from build123d import *

# Parameters (mm, degrees)
SKETCH1_W           = 110
SKETCH1_H           = 84.3
SKETCH1_R           = 1.5
SKETCH1_R_2         = 1.8
BOSS_EXTRUDE1_DEPTH = 3
BOSS_EXTRUDE2_START = 3
SKETCH2_R           = 3
SKETCH2_R_2         = 1.5
BOSS_EXTRUDE2_DEPTH = 3
FILLET1_R           = 3


with BuildPart() as part:
    # Sketch1 → Boss-Extrude1 (new body)
    with BuildSketch(Plane.XY):
        Rectangle(SKETCH1_W, SKETCH1_H)
        with Locations((51, 38.15)):
            Circle(SKETCH1_R, mode=Mode.SUBTRACT)
        with Locations(Location((-51, 38.15, 0), (0, 0, 180))):
            Circle(SKETCH1_R, mode=Mode.SUBTRACT)
        with Locations(Location((51, -38.15, 0), (0, 0, 180))):
            Circle(SKETCH1_R, mode=Mode.SUBTRACT)
        with Locations((-51, -38.15)):
            Circle(SKETCH1_R, mode=Mode.SUBTRACT)
        with Locations((-25, -17.15)):
            Circle(SKETCH1_R_2, mode=Mode.SUBTRACT)
        with Locations((-25, 2.85)):
            Circle(SKETCH1_R_2, mode=Mode.SUBTRACT)
        with Locations((10, 2.85)):
            Circle(SKETCH1_R_2, mode=Mode.SUBTRACT)
        with Locations((10, -17.15)):
            Circle(SKETCH1_R_2, mode=Mode.SUBTRACT)
    extrude(amount=BOSS_EXTRUDE1_DEPTH)

    # Sketch2 → Boss-Extrude2 (add)
    # profile 1 of 4: a face of its own
    with BuildSketch(Plane.XY.offset(BOSS_EXTRUDE2_START)):
        with Locations(Location((-51, 38.15, 0), (0, 0, 180))):
            Circle(SKETCH2_R)
        with Locations(Location((-51, 38.15, 0), (0, 0, 180))):
            Circle(SKETCH2_R_2, mode=Mode.SUBTRACT)
    # profile 2 of 4: a face of its own
    with BuildSketch(Plane.XY.offset(BOSS_EXTRUDE2_START)):
        with Locations(Location((51, 38.15, 0), (0, 0, 180))):
            Circle(SKETCH2_R)
        with Locations(Location((51, 38.15, 0), (0, 0, 180))):
            Circle(SKETCH2_R_2, mode=Mode.SUBTRACT)
    # profile 3 of 4: a face of its own
    with BuildSketch(Plane.XY.offset(BOSS_EXTRUDE2_START)):
        with Locations(Location((51, -38.15, 0), (0, 0, 180))):
            Circle(SKETCH2_R)
        with Locations(Location((51, -38.15, 0), (0, 0, 180))):
            Circle(SKETCH2_R_2, mode=Mode.SUBTRACT)
    # profile 4 of 4: a face of its own
    with BuildSketch(Plane.XY.offset(BOSS_EXTRUDE2_START)):
        with Locations(Location((-51, -38.15, 0), (0, 0, 180))):
            Circle(SKETCH2_R)
        with Locations(Location((-51, -38.15, 0), (0, 0, 180))):
            Circle(SKETCH2_R_2, mode=Mode.SUBTRACT)
    extrude(amount=BOSS_EXTRUDE2_DEPTH)

    # Fillet1
    # the kernel refuses this fillet: 3 mm, written as the material it adds along each edge
    with BuildSketch(Plane(origin=(-51, 38.15, 3), x_dir=(-1, 0, 0), z_dir=(0, 1, 0))) as fillet1_piece_1_section:
        with BuildLine():
            CenterArc((3 + FILLET1_R, FILLET1_R), FILLET1_R, 180, 90)
            Line((3, FILLET1_R), (3, 0))
            Line((3, 0), (3 + FILLET1_R, 0))
        make_face()
    fillet1_piece_1 = revolve(axis=Axis((-51, 38.15, 3), (0, 0, 1)), mode=Mode.PRIVATE)
    fillet1_piece_1 = split(fillet1_piece_1, bisect_by=Plane(origin=(-55, 38.15, 3.853016367), z_dir=(1, 0, 0)), keep=Keep.TOP, mode=Mode.PRIVATE)
    fillet1_piece_1 = split(fillet1_piece_1, bisect_by=Plane(origin=(-47.146983633, 42.15, 3.853016367), z_dir=(0, -1, 0)), keep=Keep.TOP, mode=Mode.PRIVATE)
    add(fillet1_piece_1)
    with BuildSketch(Plane(origin=(51, 38.15, 3), x_dir=(-1, 0, 0), z_dir=(0, 1, 0))) as fillet1_piece_2_section:
        with BuildLine():
            CenterArc((3 + FILLET1_R, FILLET1_R), FILLET1_R, 180, 90)
            Line((3, FILLET1_R), (3, 0))
            Line((3, 0), (3 + FILLET1_R, 0))
        make_face()
    fillet1_piece_2 = revolve(axis=Axis((51, 38.15, 3), (0, 0, 1)), mode=Mode.PRIVATE)
    fillet1_piece_2 = split(fillet1_piece_2, bisect_by=Plane(origin=(55, 38.15, 3.853016383), z_dir=(-1, 0, 0)), keep=Keep.TOP, mode=Mode.PRIVATE)
    fillet1_piece_2 = split(fillet1_piece_2, bisect_by=Plane(origin=(54.853016383, 42.15, 3.853016383), z_dir=(0, -1, 0)), keep=Keep.TOP, mode=Mode.PRIVATE)
    add(fillet1_piece_2)
    with BuildSketch(Plane(origin=(51, -38.15, 3), x_dir=(-1, 0, 0), z_dir=(0, 1, 0))) as fillet1_piece_3_section:
        with BuildLine():
            CenterArc((3 + FILLET1_R, FILLET1_R), FILLET1_R, 180, 90)
            Line((3, FILLET1_R), (3, 0))
            Line((3, 0), (3 + FILLET1_R, 0))
        make_face()
    fillet1_piece_3 = revolve(axis=Axis((51, -38.15, 3), (0, 0, 1)), mode=Mode.PRIVATE)
    fillet1_piece_3 = split(fillet1_piece_3, bisect_by=Plane(origin=(54.853016382, -42.15, 3.853016382), z_dir=(0, 1, 0)), keep=Keep.TOP, mode=Mode.PRIVATE)
    fillet1_piece_3 = split(fillet1_piece_3, bisect_by=Plane(origin=(55, -38.15, 3.853016382), z_dir=(-1, 0, 0)), keep=Keep.TOP, mode=Mode.PRIVATE)
    add(fillet1_piece_3)
    with BuildSketch(Plane(origin=(-51, -38.15, 3), x_dir=(-1, 0, 0), z_dir=(0, 1, 0))) as fillet1_piece_4_section:
        with BuildLine():
            CenterArc((3 + FILLET1_R, FILLET1_R), FILLET1_R, 180, 90)
            Line((3, FILLET1_R), (3, 0))
            Line((3, 0), (3 + FILLET1_R, 0))
        make_face()
    fillet1_piece_4 = revolve(axis=Axis((-51, -38.15, 3), (0, 0, 1)), mode=Mode.PRIVATE)
    fillet1_piece_4 = split(fillet1_piece_4, bisect_by=Plane(origin=(-47.146983624, -42.15, 3.853016376), z_dir=(0, 1, 0)), keep=Keep.TOP, mode=Mode.PRIVATE)
    fillet1_piece_4 = split(fillet1_piece_4, bisect_by=Plane(origin=(-55, -38.15, 3.853016376), z_dir=(1, 0, 0)), keep=Keep.TOP, mode=Mode.PRIVATE)
    add(fillet1_piece_4)


solid = part.part
Design review of the part built by this model. Coordinates are the model's own, in mm. A direction names the side the tool comes from. Round coordinates to 2 decimals unless told otherwise and drop trailing zeros. Write each loop counter-clockwise with the first axis right and the second up, starting at its lowest first coordinate (ties: lowest second). Pieces come first, ordered by that corner, then holes. Notation, with made-up numbers: (-5, 63) -> (11, 63) arc R30 ccw to (11, 93) -> close; hole circle Ø7 at (-9.75, -22). An arc over 180 degrees is marked (long way). One line per item, written item: value. Start each with the question number.
Q1. Add section A-A (y = 2.85). Give the boundary of the cut face in (x, z).
Q2. Add section B-B (x = -25). Give the boundary of the cut face in (y, z).
Q3. Insertion check: P1, Ø1.5, axis at x = 36, y = -29, coming from the +Z side; P2, Ø1.8, axis at x = 51, y = -38.15, coming from the +Z side. Each pin has a flat end and moves straight along its axis. Give the tip position at first contact, or say it passes through.
Q4. The part is to be moulded in two halves that separate along X. For faces 1 (the face through (49.7, 39.4, 6)), 2 (the face through (52.5, -38.2, 3)), 3 (the face through (-55, -1, 1)), 4 (the face through (-49.5, 38.1, 3)), say which applies: pulls with the +X half, pulls with the -X half, needs draft (parallel to the pull), parting line crosses it, or undercut.
Q5. Tool access review of faces 5 (the face through (-1, 1, 3)), 6 (the face through (-23.337, 2.161, 1.479)): name each direction out of +Z, -Z, +X, -X, +Y, -Y from which nothing blocks a thin tool from reaching the whole face with its end or side.
Q6. To check wall thickness, follow probe 1 along X at (y, z) = (-38.15, 2.3); probe 2 along Y at (x, z) = (10, 2); probe 3 along X at (y, z) = (-17, 2.25). State the ranges of each line that lie inside material, in increasing order.
Q7. Add section D-D (y = 38.15). Give the boundary of the cut face in (x, z).
Q8. Add section C-C (x = 51). Give the boundary of the cut face in (y, z).
Response:
1. outline: (-55, 0) -> (-26.8, 0) -> (-26.8, 3) -> (-55, 3) -> close; (-23.2, 0) -> (8.2, 0) -> (8.2, 3) -> (-23.2, 3) -> close; (11.8, 0) -> (55, 0) -> (55, 3) -> (11.8, 3) -> close
2. outline: (-42.15, 0) -> (-18.95, 0) -> (-18.95, 3) -> (-42.15, 3) -> close; (-15.35, 0) -> (1.05, 0) -> (1.05, 3) -> (-15.35, 3) -> close; (4.65, 0) -> (42.15, 0) -> (42.15, 3) -> (4.65, 3) -> close
3. P1: stops at z = 3
3. P2: passes through
4. face 1: needs draft
4. face 2: undercut
4. face 3: pulls with the -X half
4. face 4: undercut
5. face 5: +Z
5. face 6: +Z, -Z
6. probe 1: x = -55 to -52.5, -49.5 to 49.5, 52.5 to 55
6. probe 2: y = -42.15 to -18.95, -15.35 to 1.05, 4.65 to 42.15
6. probe 3: x = -55 to -26.79, -23.21 to 8.21, 11.79 to 55
7. outline: (-55, 0) -> (-52.5, 0) -> (-52.5, 6) -> (-54, 6) arc R3 cw to (-55, 3.76) -> close; (-49.5, 0) -> (49.5, 0) -> (49.5, 6) -> (48, 6) arc R3 cw to (45, 3) -> (-45, 3) arc R3 cw to (-48, 6) -> (-49.5, 6) -> close; (52.5, 0) -> (55, 0) -> (55, 3.76) arc R3 cw to (54, 6) -> (52.5, 6) -> close
8. outline: (-42.15, 0) -> (-39.65, 0) -> (-39.65, 6) -> (-41.15, 6) arc R3 cw to (-42.15, 3.76) -> close; (-36.65, 0) -> (36.65, 0) -> (36.65, 6) -> (35.15, 6) arc R3 cw to (32.15, 3) -> (-32.15, 3) arc R3 cw to (-35.15, 6) -> (-36.65, 6) -> close; (39.65, 0) -> (42.15, 0) -> (42.15, 3.76) arc R3 cw to (41.15, 6) -> (39.65, 6) -> close
